Read the model definition and answer for the solid it produces. Units are mm, in the model's axes. A direction names the side the tool comes from. Coordinates: 2 decimals unless noted, no trailing zeros. Order: outer loops, then holes, each group sorted by start corner. A loop starts at its lowest first (then second) coordinate and runs counter-clockwise, first axis right, second up. Notation, with made-up numbers: M -5.5,30 L 31.5,30 A26 ccw 31.5,56 Z; hole C -4.75,52.25 d4. An arc over 180 degrees is marked long. Use a Markdown table: item, result. Add a question column.
1) Find section B-B on z = 6.25. Write down the section's boundary in (x, y).
2) For faces 1 (the face through (-1, 0, 0)), 2 (the face through (-76, 5, -3.5)), 3 (the face through (-76, 5, 3.5)), 4 (the face through (-75.936, 2, 0)), 5 (the face through (73, 3.1, 0)), determine the directions among +Z, -Z, +X, -X, +Y, -Y from which every point of the face is accessible in a straight line to the end or side of a thin tool.
3) Find section C-C on x = 34. Write down the section's boundary in (y, z).
4) The mould has two halves that part along X. Classify faces 6 (the face through (-74.429, 10.183, 0.049)), 7 (the face through (-77, 0, 0)), 8 (the face through (-1, 3, 0)): released by +X, released by -X, zero draft, split by the parting line, or undercut.
5) Find the intervals of material crossed by probe 1 along X at (y, z) = (0.5, 3); probe 2 along Y at (x, z) = (8, 5); probe 3 along X at (y, z) = (2.25, -0.75), in increasing order. Write a range as [from, to].
6) Each of these flat-tipped pins is pushed along its axis until it touches: pin 1 Ø1.1 at (x, z) = (-77.5, 1.5) entering from +Y; pin 2 Ø0.6 at (x, z) = (75, 1.5) entering from -Y; pin 3 Ø1.5 at (x, y) = (-78, 4.5) entering from -Z. Where does it stop, or does it pass through?
7) Find section A-A on y = 6.5. Write down the section's boundary in (x, z), plus the area to 3 significant figures.
from build123d import *

# Parameters (mm, degrees)
SKETCH_1_W          = 148
SKETCH_1_H          = 20.6
EXTRUDE_1_DEPTH     = 3
EXTRUDE_START       = -1.4
SKETCH_2_W          = 4
SKETCH_2_H          = 7
EXTRUDE_2_DEPTH     = 1.5
EXTRUDE_START_2     = -10.3
EXTRUDE_4_DEPTH     = 3.5
FILLET_2_SIZE       = 1
FILLET_2_SIZE_2     = 0.5
CUT_EXTRUDE_1_REACH = 156.915
SKETCH_6_W          = 3
SKETCH_6_H          = 1.48026825
FILLET_3_R          = 0.5
FILLET_4_R          = 0.2


with BuildPart() as part:
    # 草图1 → 凸台-拉伸1 (new body)
    with BuildSketch(Plane(origin=(0, 0, 0), x_dir=(1, 0, 0), z_dir=(0, 1, 0))):
        Rectangle(SKETCH_1_W, SKETCH_1_H)
    extrude(amount=EXTRUDE_1_DEPTH)

    # 草图2 → 凸台-拉伸2 (add)
    with BuildSketch(Plane(origin=(0, 3, 0), x_dir=(1, 0, 0), z_dir=(0, 1, 0)).offset(EXTRUDE_START)):
        with Locations((74, 0)):
            Rectangle(SKETCH_2_W, SKETCH_2_H)
    extrude(amount=EXTRUDE_2_DEPTH)

    # 草图5 → 凸台-拉伸4 (add, symmetric)
    with BuildSketch(Plane.XY.offset(10.3).offset(EXTRUDE_START_2)):
        with BuildLine():
            Line((-74, 3), (-74, 9))
            ThreePointArc((-74, 9), (-74.480432289, 9.027171941), (-74.961629872, 9.02871601))
            Line((-74.961629872, 9.02871601), (-75.936491673, 3.5))
            Line((-75.936491673, 3.5), (-75.936491673, 0))
            Line((-75.936491673, 0), (-77.2, 0))
            Line((-77.2, 0), (-78.636491673, 0))
            Line((-78.636491673, 0), (-78.636491673, 1.4))
            Line((-78.636491673, 1.4), (-77.136491673, 1.4))
            Line((-77.136491673, 1.4), (-77.136491673, 3.5))
            Line((-77.136491673, 3.5), (-78.236491673, 3.5))
            Line((-78.236491673, 3.5), (-78.236491673, 4.5))
            Line((-78.236491673, 4.5), (-76.893992376, 4.98026825))
            Line((-76.893992376, 4.98026825), (-75.98900028, 10.112733474))
            ThreePointArc((-75.98900028, 10.112733474), (-74.390059228, 10.181991094), (-72.8, 10))
            Line((-72.8, 10), (-72.8, 3))
            Line((-72.8, 3), (-74, 3))
        make_face()
    extrude(amount=EXTRUDE_4_DEPTH, both=True)

    # 圆角2
    # an asymmetric fillet: 1, 0.5 mm, written as the material it takes off along each edge
    with BuildSketch(Plane(origin=(76, 3.1, -6), x_dir=(-1, 0, 0), z_dir=(0, 0, 1))) as fillet_2_piece_1:
        with BuildLine():
            Bezier((FILLET_2_SIZE, 0), (0, 0), (0, FILLET_2_SIZE_2), weights=[1, 0.707106781, 1])
            Line((0, FILLET_2_SIZE_2), (0, 0))
            Line((0, 0), (FILLET_2_SIZE, 0))
        make_face()
    extrude(amount=12, mode=Mode.SUBTRACT)

    # 切除-拉伸1: up to this plane
    cut_extrude_1_end = Plane(origin=(-61993.202735843, -351139.85584642, 3.5), z_dir=(0.984807753012209, -0.17364817766692522, 0))
    # 草图6 → 切除-拉伸1 (cut, up to the surface)
    with BuildSketch(Plane.ZY.offset(78.236491673), mode=Mode.PRIVATE) as cut_extrude_1_sk1:
        with Locations((0, 4.240134125)):
            Rectangle(SKETCH_6_W, SKETCH_6_H)
    cut_extrude_1_tool1 = split(extrude(cut_extrude_1_sk1.sketch, amount=-CUT_EXTRUDE_1_REACH, mode=Mode.PRIVATE), bisect_by=cut_extrude_1_end, keep=Keep.BOTH, mode=Mode.PRIVATE)
    add(cut_extrude_1_tool1.solids().sort_by_distance((-78.236492, 4.240134, 0))[0], mode=Mode.SUBTRACT)

    # 圆角3
    fillet_3_edges = [part.edges().sort_by_distance(p)[0] for p in [
        (-74, 3, -6.9),
        (-74, 3, 6.9),
        (-74.961629872, 9.02871601, 0),
        (-74, 9, 0),
        (-72.8, 10, 0),
        (-75.98900028, 10.112733474, 0),
        (-78.236491673, 4.5, 2.5),
        (-78.636491673, 1.4, 0),
        (-78.236491673, 4.5, -2.5),
    ]]
    fillet(fillet_3_edges, radius=FILLET_3_R)

    # 圆角4
    fillet_4_edges = [part.edges().sort_by_distance(p)[0] for p in [
        (-78.236491673, 3.5, 2.5),
        (-78.236491673, 3.5, -2.5),
    ]]
    fillet(fillet_4_edges, radius=FILLET_4_R)


solid = part.part
Check result:
| question | item | result |
|---|---|---|
| 1 | outline | M -74,0 L 74,0 L 74,3 L -73.5,3 A0.5 ccw -74,2.5 Z |
| 2 | face 1 | +Z, -Z, +X, -X, -Y |
| 2 | face 2 | -Z, -X, +Y |
| 2 | face 3 | +Z, -X, +Y |
| 2 | face 4 | +Z, -Z, -Y |
| 2 | face 5 | +Z, -Z, +X, +Y |
| 3 | outline | M 0,-10.3 L 3,-10.3 L 3,10.3 L 0,10.3 Z |
| 4 | face 6 | split by the parting line |
| 4 | face 7 | zero draft |
| 4 | face 8 | undercut |
| 5 | probe 1 | x = [-78.64, -75.94], [-74, 74] |
| 5 | probe 2 | y = [0, 3] |
| 5 | probe 3 | x = [-77.14, -75.94], [-74, 76] |
| 6 | pin 1 | stops at y = 4.96 |
| 6 | pin 2 | stops at y = 1.6 |
| 6 | pin 3 | stops at z = -3.5 |
| 7 | outline | M -76.63,-3.5 L -75.41,-3.5 L -75.41,3.5 L -76.63,3.5 Z; M -74,-3.5 L -72.8,-3.5 L -72.8,3.5 L -74,3.5 Z |
| 7 | area | 16.9 mm2 |
